Design review of the part built by this model. Coordinates are the model's own, in mm. Give positions to 0.01 mm unless a question says otherwise; leave off trailing zeros. Write each loop counter-clockwise with the first axis right and the second up, starting at its lowest first coordinate (ties: lowest second). Pieces come first, ordered by that corner, then holes. Notation, with made-up numbers: M 44,57.25 L 85,57.25 A34 cw 85,88.25 Z; hole C 36,-5 d2. An arc over 180 degrees is marked long. Answer in a Markdown table with one row per item.
Autodesk Inventor part; units mm, degrees
ref_plane "YZ Plane" through (0, 0, 0) normal (1, 0, 0) x (0, 1, 0)
ref_plane "XZ Plane" through (0, 0, 0) normal (0, 1, 0) x (-1, 0, 0)
ref_plane "XY Plane" through (0, 0, 0) normal (0, 0, 1) x (1, 0, 0)
sketch "Sketch1" plane through (0, 0, 0) normal (0, 0, 1) x (1, 0, 0)
  line L0 (0, 0) -> (66.04, 0)
  line L1 (66.04, 0) -> (66.04, 58.42)
  line L2 (66.04, 58.42) -> (0, 58.42)
  line L3 (0, 58.42) -> (0, 0)
  dimension "d0" = 66.04
  dimension "d1" = 58.42
extrude "Extrusion1" add sketch "Sketch1" along normal blind 22.86
sketch "Sketch2" plane through (0, 0, 22.86) normal (0, 0, 1) x (1, 0, 0)
  line L0 (0, 0) -> (66.04, 0)
  point P0 (33.02, 49.7501)
  point P1 (33.02, 8.221)
  point P2 (33.02, 0)
  point P3 (33.02, 0)
hole "Hole1" at (33.02, 49.7501, 22.86) at (33.02, 8.221, 22.86) direction (0, 0, -1) diameter 6.35 end through all
properties part number "+5V Regulator"
1) Add section A-A (x = 33.02). Write out the cut boundary in (y, z), and give its area (3 significant figures).
Geometry says:
| item | result |
|---|---|
| outline | M 0,0 L 5.05,0 L 5.05,22.86 L 0,22.86 Z; M 11.4,0 L 46.58,0 L 46.58,22.86 L 11.4,22.86 Z; M 52.93,0 L 58.42,0 L 58.42,22.86 L 52.93,22.86 Z |
| area | 1,050 mm^2 |
2) The part is to be moulded in two halves that separate along X. For faces 1 (the face through (0, 30, 11)), 2 (the face through (36.12, 8.91, 11.27)), 3 (the face through (34.24, 46.82, 11.27)), 4 (the face through (33, 30, 22.86)), say which applies: released by +X, released by -X, zero draft, split by the parting line, or undercut.
Geometry says:
| item | result |
|---|---|
| face 1 | released by -X |
| face 2 | undercut |
| face 3 | undercut |
| face 4 | zero draft |
3) Add section B-B (y = 50). Write out the cut boundary in (x, z).
Geometry says:
| item | result |
|---|---|
| outline | M 0,0 L 29.85,0 L 29.85,22.86 L 0,22.86 Z; M 36.19,0 L 66.04,0 L 66.04,22.86 L 36.19,22.86 Z |
4) To check wall thickness, follow probe 1 along Y at (x, z) = (33.02, 16.5); probe 2 along X at (y, z) = (7, 5.25); probe 3 along X at (y, z) = (48, 19). State the ranges of each line that lie inside material, in increasing order. Write a range as [from, to].
Geometry says:
| item | result |
|---|---|
| probe 1 | [0, 5.05], [11.4, 46.58], [52.93, 58.42] |
| probe 2 | [0, 30.09], [35.95, 66.04] |
| probe 3 | [0, 30.37], [35.67, 66.04] |
5) Add section C-C (z = 21). Write out the cut boundary in (x, y) (3 decimals).
Geometry says:
| item | result |
|---|---|
| outline | M 0,0 L 66.04,0 L 66.04,58.42 L 0,58.42 Z; hole C 33.02,8.221 d6.35; hole C 33.02,49.75 d6.35 |
